from build123d import *

# Parameters (mm, degrees)
SKETCH1_R           = 20
BOSS_EXTRUDE1_DEPTH = 15
FILLET1_R           = 10
SKETCH2_R           = 14
CUT_EXTRUDE1_DEPTH  = 13
SKETCH4_R           = 10.4
CUT_EXTRUDE3_DEPTH  = 11
SKETCH3_R           = 18.4
CUT_EXTRUDE4_DEPTH  = 10


with BuildPart() as part:
    # Sketch1 → Boss-Extrude1 (new body)
    with BuildSketch(Plane.XY):
        Circle(SKETCH1_R)
    extrude(amount=BOSS_EXTRUDE1_DEPTH)

    # Fillet1
    fillet1_edges = [part.edges().sort_by_distance(p)[0] for p in [
        (-20, 0, 0),
    ]]
    fillet(fillet1_edges, radius=FILLET1_R)

    # Sketch2 → Cut-Extrude1 (cut)
    with BuildSketch(Plane.XY.offset(15)):
        Circle(SKETCH2_R)
    extrude(amount=-CUT_EXTRUDE1_DEPTH, mode=Mode.SUBTRACT)

    # Sketch4 → Cut-Extrude3 (cut)
    with BuildSketch(Plane(origin=(0, 0, 0), x_dir=(-1, 0, 0), z_dir=(0, 0, -1))):
        with Locations(Location((0, 0, 0), (0, 0, 180))):
            Circle(SKETCH4_R)
    extrude(amount=-CUT_EXTRUDE3_DEPTH, mode=Mode.SUBTRACT)

    # Sketch3 → Cut-Extrude4 (cut)
    with BuildSketch(Plane.XY.offset(15)):
        Circle(SKETCH3_R)
    extrude(amount=-CUT_EXTRUDE4_DEPTH, mode=Mode.SUBTRACT)


solid = part.part
Check sheet for the modelled part. Datum: model origin and axes. Units: mm. Round coordinates to 2 decimals unless told otherwise and drop trailing zeros. One line per item, written item: value.
(1) Depth check by flat-ended pin: pin 1 Ø2 at (x, y) = (-14.5, -8.5) entering from +Z; pin 2 Ø3 at (x, z) = (13, 11) entering from +Y; pin 3 Ø6 at (y, z) = (-10.5, 10.5) entering from +X. Enter the tip coordinate at first touch or a pass-through.
Computed values:
pin 1: stops at z = 5
pin 2: stops at y = 16.36
pin 3: stops at x = 18.54
(2) Release check for a two-part mould opening along X. For faces 1 (the face through (18, -6, 15)), 2 (the face through (9.92, -3.12, 0.99)), 3 (the face through (-4.336, -19.524, 12.465)), 4 (the face through (-14.6, -11.2, 10.1)) record: +X half, -X half, draft (parallel to the pull), parting line (faces both ways), or undercut.
Computed values:
face 1: draft
face 2: undercut
face 3: parting line
face 4: undercut
(3) Thickness scan on line 1 (Y direction, x = 0, z = 11.75); line 2 (X direction, y = 16, z = 8); line 3 (Y direction, x = 0, z = 0.85). Record the ranges inside material, lowest first.
Computed values:
line 1: y = -20 to -18.4, 18.4 to 20
line 2: x = -11.66 to -9.09, 9.09 to 11.66
line 3: y = -14.03 to -10.4, 10.4 to 14.03
